```python
from build123d import *

# Parameters (mm, degrees)
F0_W     = 355.6
F0_H     = 355.6
F1_DEPTH = 25.4


with BuildPart() as f1:
    # F0 (on Front) → F1 (new body)
    with BuildSketch(Plane.XZ):
        Rectangle(F0_W, F0_H)
        Polygon((76.372818, 114.3), (114.3, 114.3), (114.3, 76.372818), (149.340147, 61.858714), (134.826043, 26.818567), (161.64461, 0), (134.826043, -26.818567), (149.340147, -61.858714), (114.3, -76.372818), (114.3, -114.3), (76.372818, -114.3), (61.858714, -149.340147), (26.818567, -134.826043), (0, -161.64461), (-26.818567, -134.826043), (-61.858714, -149.340147), (-76.372818, -114.3), (-114.3, -114.3), (-114.3, -76.372818), (-149.340147, -61.858714), (-134.826043, -26.818567), (-161.64461, 0), (-134.826043, 26.818567), (-149.340147, 61.858714), (-114.3, 76.372818), (-114.3, 114.3), (-76.372818, 114.3), (-61.858714, 149.340147), (-26.818567, 134.826043), (0, 161.64461), (26.818567, 134.826043), (61.858714, 149.340147), align=None, mode=Mode.SUBTRACT)
    extrude(amount=F1_DEPTH)


solid = f1.part
```
CAD build for the part. Positions are in the model's coordinates, mm. A direction names the side the tool comes from. Coordinates: 2 decimals unless noted, no trailing zeros. Write each loop counter-clockwise with the first axis right and the second up, starting at its lowest first coordinate (ties: lowest second). Pieces come first, ordered by that corner, then holes.
(1) Drill centre lines: probe 1 along X at (y, z) = (-19.5, 88); probe 2 along Z at (x, y) = (-140, -4.5); probe 3 along X at (y, z) = (-21.5, -147.5). Where is each one in solid material? Low to high.
(2) Cut at A-A, the plane z = -91. List the corners of the cut face in (x, y).
(3) Cut at B-B, the plane x = -92.5. List the corners of the cut face in (y, z), and give its area (3 significant figures).
(4) 3-axis set-ups, long thin cutter, end or side, ignore diameter. For faces 1 (the face through (148.423, -12.522, -13.222)), 2 (the face through (-2, -13, 177.8)): which of +Z, -Z, +X, -X, +Y, -Y reach the whole face in a straight line?
(5) Two-plate mould, pull along X, no slides. Class faces 3 (the face through (-2, -13, -177.8)), 4 (the face through (-114.3, -13, -96)): +X half, -X half, draft (parallel to the pull), parting line (faces both ways), or undercut.
Geometry says:
1. probe 1: x = -177.8 to -114.3, 114.3 to 177.8
1. probe 2: z = -177.8 to -65.73, -39.31 to -21.64, 21.64 to 39.31, 65.73 to 177.8
1. probe 3: x = -177.8 to -62.62, -57.42 to -14.14, 14.14 to 57.42, 62.62 to 177.8
2. outline: (-177.8, -25.4) - (-114.3, -25.4) - (-114.3, 0) - (-177.8, 0) - close; (114.3, -25.4) - (177.8, -25.4) - (177.8, 0) - (114.3, 0) - close
3. outline: (-25.4, -177.8) - (0, -177.8) - (0, -114.3) - (-25.4, -114.3) - close; (-25.4, 114.3) - (0, 114.3) - (0, 177.8) - (-25.4, 177.8) - close
3. area: 3,230 mm2
4. face 1: +Y, -Y
4. face 2: +Z, +X, -X, +Y, -Y
5. face 3: draft
5. face 4: undercut
